The model under review builds one solid part; all positions refer to its coordinate system, in mm. A direction names the side the tool comes from. Round coordinates to 2 decimals unless told otherwise and drop trailing zeros. Order: outer loops, then holes, each group sorted by start corner. A loop starts at its lowest first (then second) coordinate and runs counter-clockwise, first axis right, second up.
```python
from build123d import *

# Parameters (mm, degrees)
EXTRUDE_THIN1_DEPTH     = 50.8
BODY_MOVE_COPY1_DEPTH   = 50.8
BODY_MOVE_COPY1_2_DEPTH = 50.8


# Read off the part's stored shape, not the designer's step: Body-Move/Copy1
with BuildPart() as part:
    # Sketch1 → Extrude-Thin1 (new body)
    with BuildSketch(Plane(origin=(0, 0, 0), x_dir=(0, 0, -1), z_dir=(1, 0, 0))):
        with BuildLine():
            Line((21.494042733, 166.084405055), (740.806573551, 99.245982925))
            ThreePointArc((740.806573551, 99.245982925), (782.028393343, 52.126153258), (737.113874036, 8.511904093))
            Line((737.113874036, 8.511904093), (456.21754645, 5.336904093))
            ThreePointArc((456.21754645, 5.336904093), (455.703672415, 5.334), (455.189798379, 5.336904093))
            Line((455.189798379, 5.336904093), (174.293470793, 8.511904093))
            ThreePointArc((174.293470793, 8.511904093), (160.890624168, 10.691261229), (148.729118574, 16.731433154))
            Line((148.729118574, 16.731433154), (3.898404857, 118.142990663))
            ThreePointArc((3.898404857, 118.142990663), (-5.748493412, 148.883347208), (21.494042733, 166.084405055))
        make_face()
        with BuildLine():
            Line((20.812530817, 158.75), (740.125061635, 91.91157787))
            ThreePointArc((740.125061635, 91.91157787), (774.668486042, 52.425687087), (737.0306207, 15.877433597))
            Line((737.0306207, 15.877433597), (456.134293115, 12.702433597))
            ThreePointArc((456.134293115, 12.702433597), (455.703672415, 12.7), (455.273051714, 12.702433597))
            Line((455.273051714, 12.702433597), (174.376724129, 15.877433597))
            ThreePointArc((174.376724129, 15.877433597), (163.145288409, 17.703710527), (152.954082604, 22.765307113))
            Line((152.954082604, 22.765307113), (8.123368888, 124.176864621))
            ThreePointArc((8.123368888, 124.176864621), (1.166471097, 146.345390976), (20.812530817, 158.75))
        make_face(mode=Mode.SUBTRACT)
    extrude(amount=EXTRUDE_THIN1_DEPTH)

    # Body-Move/Copy1 outline → Body-Move/Copy1 (cut)
    with BuildSketch(Plane.YZ):
        with BuildLine():
            ThreePointArc((166.084405055, -21.494042733), (164.537643621, -9.833229454), (158.082054122, 0))
            ThreePointArc((158.082054122, 0), (155.175079711, -2.417399882), (151.952776868, -4.395046666))
            ThreePointArc((151.952776868, -4.395046666), (157.382799095, -11.762737128), (158.75, -20.812530817))
            Line((158.75, -20.812530817), (91.91157787, -740.125061635))
            ThreePointArc((91.91157787, -740.125061635), (52.425687087, -774.668486042), (15.877433597, -737.0306207))
            Line((15.877433597, -737.0306207), (12.702433597, -456.134293115))
            ThreePointArc((12.702433597, -456.134293115), (12.7, -455.703672414), (12.702433597, -455.273051714))
            Line((12.702433597, -455.273051714), (15.877433597, -174.376724129))
            ThreePointArc((15.877433597, -174.376724129), (17.703710527, -163.145288409), (22.765307113, -152.954082604))
            Line((22.765307113, -152.954082604), (124.176864621, -8.123368888))
            ThreePointArc((124.176864621, -8.123368888), (125.769201584, -6.144494274), (127.610645261, -4.395046667))
            ThreePointArc((127.610645261, -4.395046667), (124.388342418, -2.417399882), (121.481368008, 0))
            ThreePointArc((121.481368008, 0), (119.717275174, -1.867931777), (118.142990663, -3.898404857))
            Line((118.142990663, -3.898404857), (16.731433154, -148.729118574))
            ThreePointArc((16.731433154, -148.729118574), (10.691261229, -160.890624168), (8.511904093, -174.293470793))
            Line((8.511904093, -174.293470793), (5.336904093, -455.189798379))
            ThreePointArc((5.336904093, -455.189798379), (5.334, -455.703672415), (5.336904093, -456.21754645))
            Line((5.336904093, -456.21754645), (8.511904093, -737.113874036))
            ThreePointArc((8.511904093, -737.113874036), (52.126153258, -782.028393343), (99.245982925, -740.806573551))
            Line((99.245982925, -740.806573551), (166.084405055, -21.494042733))
        make_face()
        with BuildLine():
            ThreePointArc((127.610645261, 4.395046667), (139.781711065, 0), (151.952776868, 4.395046666))
            ThreePointArc((151.952776868, 4.395046666), (139.781711065, 7.366), (127.610645261, 4.395046667))
        make_face()
    extrude(amount=BODY_MOVE_COPY1_DEPTH, mode=Mode.SUBTRACT)

    # Body-Move_Copy1 2 outline → Body-Move_Copy1 2 (add)
    with BuildSketch(Plane.YZ):
        with BuildLine():
            ThreePointArc((158.082054122, 0), (164.537643621, 9.833229454), (166.084405055, 21.494042733))
            Line((166.084405055, 21.494042733), (99.245982925, 740.806573551))
            ThreePointArc((99.245982925, 740.806573551), (52.126153258, 782.028393343), (8.511904093, 737.113874036))
            Line((8.511904093, 737.113874036), (5.336904093, 456.21754645))
            ThreePointArc((5.336904093, 456.21754645), (5.334, 455.703672415), (5.336904093, 455.189798379))
            Line((5.336904093, 455.189798379), (8.511904093, 174.293470793))
            ThreePointArc((8.511904093, 174.293470793), (10.691261229, 160.890624168), (16.731433154, 148.729118574))
            Line((16.731433154, 148.729118574), (118.142990663, 3.898404857))
            ThreePointArc((118.142990663, 3.898404857), (119.717275174, 1.867931777), (121.481368008, 0))
            ThreePointArc((121.481368008, 0), (124.388342418, 2.417399882), (127.610645261, 4.395046667))
            ThreePointArc((127.610645261, 4.395046667), (125.769201584, 6.144494274), (124.176864621, 8.123368888))
            Line((124.176864621, 8.123368888), (22.765307113, 152.954082604))
            ThreePointArc((22.765307113, 152.954082604), (17.703710527, 163.145288409), (15.877433597, 174.376724129))
            Line((15.877433597, 174.376724129), (12.702433597, 455.273051714))
            ThreePointArc((12.702433597, 455.273051714), (12.7, 455.703672415), (12.702433597, 456.134293115))
            Line((12.702433597, 456.134293115), (15.877433597, 737.0306207))
            ThreePointArc((15.877433597, 737.0306207), (52.425687087, 774.668486042), (91.91157787, 740.125061635))
            Line((91.91157787, 740.125061635), (158.75, 20.812530817))
            ThreePointArc((158.75, 20.812530817), (157.382799095, 11.762737128), (151.952776868, 4.395046666))
            ThreePointArc((151.952776868, 4.395046666), (155.175079711, 2.417399882), (158.082054122, 0))
        make_face()
        with BuildLine():
            ThreePointArc((127.610645261, -4.395046667), (139.781711065, -7.366), (151.952776868, -4.395046666))
            ThreePointArc((151.952776868, -4.395046666), (139.781711065, 0), (127.610645261, -4.395046667))
        make_face()
    extrude(amount=BODY_MOVE_COPY1_2_DEPTH)


solid = part.part
```
(1) To check wall thickness, follow probe 1 along Y at (x, z) = (44, 162.5); probe 2 along Y at (x, z) = (11, 111); probe 3 along Z at (x, y) = (3, 37). State the ranges of each line that lie inside material, in increasing order.
Data:
probe 1: y = 10.21 to 17.92, 145.58 to 152.98
probe 2: y = 43.15 to 52.14, 150.37 to 157.77
probe 3: z = 119.78 to 132.62, 770.71 to 778.78
(2) Draft analysis for pull direction Z (two halves, no side actions). For faces 1 (the flat face through (25.044, 66.727, 77.328)), 2 (the flat face through (50.8, 127, 389)), 3 (the cylindrical face through (25.044, 51.617, 774.627)), state which applies: pulls with the +Z half, pulls with the -Z half, needs draft (parallel to the pull), parting line crosses it, or undercut.
Data:
face 1: pulls with the -Z half
face 2: needs draft
face 3: undercut
(3) Insertion check: pin 1 (1.5 mm diameter, centred on x = 8.5, y = 30.5, fed in from +Z); pin 2 (5 mm diameter, centred on x = 21, z = 174, fed in from +Y); pin 3 (5 mm diameter, centred on x = 41.5, y = 61, fed in from +Z). Each pin has a flat end and moves straight along its axis. Give the tip position at first contact, or say it passes through.
Data:
pin 1: stops at z = 775.98
pin 2: stops at y = 152.15
pin 3: stops at z = 781.84
(4) Consider section B-B (z = 263). Write out the cut boundary in (x, y), and give its area (3 significant figures).
Data:
outline: (0, 7.51) - (50.8, 7.51) - (50.8, 14.88) - (0, 14.88) - close; (0, 136.25) - (50.8, 136.25) - (50.8, 143.64) - (0, 143.64) - close
area: 750 mm2
(5) For faces 4 (the flat face through (25, 74.2, 79.5)), 5 (the cylindrical face through (25.044, 10.633, 161.072)), list the 3-axis set-ups (+Z, -Z, +X, -X, +Y, -Y) from which the entire face can be reached by the end or side of a thin tool; tool diameter is ignored.
Data:
face 4: +X, -X
face 5: -Z, +X, -X, -Y
(6) Consider section A-A (y = 142.5). Write out the cut boundary in (x, z), and give its area (3 significant figures).
Data:
outline: (0, -7.23) - (50.8, -7.23) - (50.8, 0.19) - (0, 0.19) - close; (0, 195.69) - (50.8, 195.69) - (50.8, 275.31) - (0, 275.31) - close
area: 4,420 mm2
(7) Consider section C-C (x = 18). Write out the cut boundary in (y, z) (3 decimals), and give its area (3 significant figures).
Data:
outline: (5.337, 455.19) - (8.512, 174.293) arc R45.466 ccw to (16.731, 148.729) - (118.143, 3.898) arc R26.416 ccw to (166.084, 21.494) - (99.246, 740.807) arc R45.466 ccw to (8.512, 737.114) - (5.337, 456.218) arc R45.466 ccw to start; hole (12.702, 455.273) - (15.877, 174.377) arc R38.1 ccw to (22.765, 152.954) - (124.177, 8.123) arc R19.05 ccw to (158.75, 20.813) - (91.912, 740.125) arc R38.1 ccw to (15.877, 737.031) - (12.702, 456.134) arc R38.1 ccw to start
area: 12,300 mm2
